from build123d import *

# Parameters (mm, degrees)
BOSS_EXTRUDE1_DEPTH      = 3
BOSS_EXTRUDE2_DEPTH      = 1
CUT_EXTRUDE1_START       = -3
CUT_EXTRUDE1_OUTLINE_R   = 1.55
CUT_EXTRUDE1_OUTLINE_R_2 = 1
CUT_EXTRUDE1_DEPTH       = 3


# Read off the part's stored shape, not the designer's step: Cut-Extrude1
with BuildPart() as part:
    # Sketch1 → Boss-Extrude1 (new body)
    with BuildSketch(Plane.XY):
        with BuildLine():
            ThreePointArc((0, 7.5), (2.196699141, 2.196699141), (7.5, 0))
            ThreePointArc((7.5, 0), (12.803300859, 2.196699141), (15, 7.5))
            Line((15, 7.5), (15, 85))
            Line((15, 85), (0, 85))
            Line((0, 85), (0, 7.5))
        make_face()
        with BuildLine():
            Line((2.49254211, 10.759753131), (5, 24.25))
            ThreePointArc((5, 24.25), (7.5, 26.75), (10, 24.25))
            Line((10, 24.25), (12.49254211, 10.782552099))
            ThreePointArc((12.49254211, 10.782552099), (7.513622348, 1.525015529), (2.49254211, 10.759753131))
        make_face(mode=Mode.SUBTRACT)
    extrude(amount=BOSS_EXTRUDE1_DEPTH)

    # Sketch1_3 → Boss-Extrude2 (add)
    with BuildSketch(Plane.XY):
        with BuildLine():
            ThreePointArc((10, 24.25), (7.5, 26.75), (5, 24.25))
            Line((5, 24.25), (2.49254211, 10.759753131))
            ThreePointArc((2.49254211, 10.759753131), (7.513622348, 1.525015529), (12.49254211, 10.782552099))
            Line((12.49254211, 10.782552099), (10, 24.25))
        make_face()
    extrude(amount=BOSS_EXTRUDE2_DEPTH)

    # Cut-Extrude1 outline → Cut-Extrude1 (cut)
    with BuildSketch(Plane.XY.offset(3).offset(CUT_EXTRUDE1_START)):
        with BuildLine():
            ThreePointArc((3.029881724, 83.522295459), (5.145983851, 84.620997681), (7.5, 85))
            Line((7.5, 85), (0, 85))
            Line((0, 85), (0, 28.334866171))
            ThreePointArc((0, 28.334866171), (0.657652773, 31.727350556), (2.173846049, 34.832606652))
            ThreePointArc((2.173846049, 34.832606652), (2.882144346, 37.314502111), (3.029881724, 39.891256895))
            Line((3.029881724, 39.891256895), (3.029881724, 83.522295459))
        make_face()
        with BuildLine():
            ThreePointArc((12.826153951, 34.832606652), (14.342347227, 31.727350556), (15, 28.334866171))
            Line((15, 28.334866171), (15, 85))
            Line((15, 85), (7.5, 85))
            ThreePointArc((7.5, 85), (9.854016149, 84.620997681), (11.970118276, 83.522295459))
            Line((11.970118276, 83.522295459), (11.970118276, 39.891256895))
            ThreePointArc((11.970118276, 39.891256895), (12.117855654, 37.314502111), (12.826153951, 34.832606652))
        make_face()
        with Locations((7.5, 7.5)):
            Circle(CUT_EXTRUDE1_OUTLINE_R)
        with Locations((7.5, 82.5)):
            Circle(CUT_EXTRUDE1_OUTLINE_R_2)
    extrude(amount=CUT_EXTRUDE1_DEPTH, mode=Mode.SUBTRACT)


solid = part.part
Work out the finished part from the listing and answer in its coordinate system (mm). A direction names the side the tool comes from. Round coordinates to 2 decimals unless told otherwise and drop trailing zeros. Write each loop counter-clockwise with the first axis right and the second up, starting at its lowest first coordinate (ties: lowest second). Pieces come first, ordered by that corner, then holes.
1) A tool of negligible diameter and unlimited length cuts with its end or side. For faces 4 (the cylindrical face through (8.215, 6.125, 0.493)), 5 (the flat face through (11.97, 62, 1)), 6 (the flat face through (11.23, 17.61, 1.99)), 7 (the flat face through (3.03, 61, 1)), from which of +Z, -Z, +X, -X, +Y, -Y can it reach the whole face along a straight path? Write none if from no direction.
2) Straight lines are drawn through the part: line 1 (Y direction, x = 7.5, z = 0.6); line 2 (X direction, y = 82.5, z = 1.35); line 3 (X direction, y = 7.5, z = 2.45) (3 decimals). For each, find the intervals that lie inside material, in ascending order.
3) A cutting plane is placed at B-B (y = 19.5). Give the vertices of the cut face in (x, z), plus the area to 3 significant figures.
4) A cutting plane is placed at C-C (y = 68.5). Give the vertices of the cut face in (x, z), plus the area to 3 significant figures.
5) Given pin 1 Ø1.5 at (x, z) = (10, 1) entering from +Y; pin 2 Ø1.5 at (y, z) = (64.5, 1) entering from -X, each flat-ended and moving along its own axis, determine where each tip first touches the part or whether it passes through.
6) A cutting plane is placed at A-A (z = 2.2). Give the number of separate pieces and of enclosed holes in the cut face, plus the area to 3 significant figures.
7) The mould has two halves that part along X. Classify faces 1 (the cylindrical face through (7.69, 1.53, 1.99)), 2 (the flat face through (0, 18, 1)), 3 (the cylindrical face through (14.33, 31.77, 1.48)): pulls with the +X half, pulls with the -X half, needs draft (parallel to the pull), parting line crosses it, or undercut.
Completed:
1. face 4: +Z, -Z
1. face 5: +Z, -Z, +X, +Y
1. face 6: +Z
1. face 7: +Z, -Z, -X, +Y
2. line 1: y = 0 to 5.95, 9.05 to 81.5, 83.5 to 85
2. line 2: x = 3.03 to 6.5, 8.5 to 11.97
2. line 3: x = 0 to 1.525, 13.475 to 15
3. outline: (0, 0) - (15, 0) - (15, 3) - (10.88, 3) - (10.88, 1) - (4.12, 1) - (4.12, 3) - (0, 3) - close
3. area: 31.5 mm2
4. outline: (3.03, 0) - (11.97, 0) - (11.97, 3) - (3.03, 3) - close
4. area: 26.8 mm2
5. pin 1: stops at y = 84.79
5. pin 2: stops at x = 3.03
6. separate pieces: 1
6. enclosed holes: 2
6. area: 728 mm2
7. face 1: undercut
7. face 2: pulls with the -X half
7. face 3: pulls with the +X half
